```python
from build123d import *

# Parameters (mm, degrees)
SALIENTE_EXTRUIR1_DEPTH = 40
REDONDEO3_R             = 4
CROQUIS4_R              = 2.25
CORTAR_EXTRUIR3_DEPTH   = 70.282032303
CROQUIS5_R              = 4.15
CORTAR_EXTRUIR4_DEPTH   = 25
CORTAR_EXTRUIR6_DEPTH   = 1
CROQUIS9_R              = 2.65
CORTAR_EXTRUIR7_DEPTH   = 24
SALIENTE_EXTRUIR2_DEPTH = 5
SALIENTE_EXTRUIR3_START = 6
CROQUIS12_W             = 6
CROQUIS12_H             = 1.5
SALIENTE_EXTRUIR3_DEPTH = 6


with BuildPart() as part:
    # Croquis1 → Saliente-Extruir1 (new body)
    with BuildSketch(Plane(origin=(0, 0, 0), x_dir=(1, 0, 0), z_dir=(0, 1, 0))):
        Polygon((0, 0), (40, 0), (40, 20), (20, 20), (20, 40), (0, 40), align=None)
    extrude(amount=SALIENTE_EXTRUIR1_DEPTH)

    # Redondeo3
    redondeo3_edges = [part.edges().sort_by_distance(p)[0] for p in [
        (40, 40, -10),
        (0, 20, -40),
        (20, 20, -40),
        (20, 20, -20),
        (40, 20, -20),
        (40, 20, 0),
        (0, 20, 0),
        (30, 40, -20),
        (20, 40, -30),
        (10, 40, -40),
        (0, 40, -20),
        (20, 40, 0),
    ]]
    fillet(redondeo3_edges, radius=REDONDEO3_R)

    # Croquis4 → Cortar-Extruir3 (cut, through all)
    with BuildSketch(Plane(origin=(0, 40, 0), x_dir=(1, 0, 0), z_dir=(0, 1, 0))):
        with Locations(Location((10, 30, 0), (0, 0, 270))):
            Circle(CROQUIS4_R)
        with Locations(Location((10, 10, 0), (0, 0, 270))):
            Circle(CROQUIS4_R)
    extrude(amount=-CORTAR_EXTRUIR3_DEPTH, mode=Mode.SUBTRACT)

    # Croquis5 → Cortar-Extruir4 (cut)
    with BuildSketch(Plane(origin=(40, 0, 0), x_dir=(0, 0, -1), z_dir=(1, 0, 0))):
        with Locations((10, 30)):
            Circle(CROQUIS5_R)
    extrude(amount=-CORTAR_EXTRUIR4_DEPTH, mode=Mode.SUBTRACT)

    # Croquis8 → Cortar-Extruir6 (cut)
    with BuildSketch(Plane(origin=(0, 40, 0), x_dir=(1, 0, 0), z_dir=(0, 1, 0))):
        Polygon((12.421293342, 18.801682692), (12.421293342, 18.692307692), (8.267447188, 18.692307692), (8.267447188, 18), (7.652062573, 18), (7.652062573, 18.692307692), (6.267447188, 18.692307692), (6.267447188, 19.230769231), (7.652062573, 19.230769231), (7.652062573, 22.076923077), align=None)
        Polygon((8.267447188, 19.230769231), (10.873216419, 19.230769231), (8.267447188, 21.019230769), align=None, mode=Mode.SUBTRACT)
    extrude(amount=-CORTAR_EXTRUIR6_DEPTH, mode=Mode.SUBTRACT)

    # Croquis9 → Cortar-Extruir7 (cut)
    with BuildSketch(Plane.XY):
        with Locations((26, 20)):
            Circle(CROQUIS9_R)
    extrude(amount=-CORTAR_EXTRUIR7_DEPTH, mode=Mode.SUBTRACT)

    # Croquis11 → Saliente-Extruir2 (add)
    with BuildSketch(Plane(origin=(0, 40, 0), x_dir=(1, 0, 0), z_dir=(0, 1, 0))):
        with BuildLine():
            Line((30, 18.5), (39.122498999, 18.5))
            ThreePointArc((39.122498999, 18.5), (39.774254628, 17.324764885), (40, 16))
            Line((40, 16), (40, 4))
            ThreePointArc((40, 4), (39.774254628, 2.675235115), (39.122498999, 1.5))
            Line((39.122498999, 1.5), (30, 1.5))
            Line((30, 1.5), (30, 18.5))
        make_face()
    extrude(amount=-SALIENTE_EXTRUIR2_DEPTH)

    # Croquis12 → Saliente-Extruir3 (add)
    with BuildSketch(Plane(origin=(0, 40, 0), x_dir=(1, 0, 0), z_dir=(0, 1, 0)).offset(SALIENTE_EXTRUIR3_START)):
        with Locations((33, 2.25)):
            Rectangle(CROQUIS12_W, CROQUIS12_H)
        with BuildLine():
            Line((30, 18.5), (39.122498999, 18.5))
            ThreePointArc((39.122498999, 18.5), (39.57724661, 17.789778391), (39.872983346, 17))
            Line((39.872983346, 17), (30, 17))
            Line((30, 17), (30, 18.5))
        make_face()
    extrude(amount=-SALIENTE_EXTRUIR3_DEPTH)


solid = part.part
```
Here's how the part is built. I have some questions about the finished solid (model axes, mm). A direction names the side the tool comes from. Coordinates: 2 decimals unless noted, no trailing zeros. Order: outer loops, then holes, each group sorted by start corner. A loop starts at its lowest first (then second) coordinate and runs counter-clockwise, first axis right, second up.
1) Imagine slicing it at D-D on x = 26.5. List the corners of the cut face in (y, z) for me, and give its area (3 significant figures).
2) I need wall thicknesses on line 1 (X direction, y = 20, z = -10.25); line 2 (X direction, y = 16.5, z = -10); line 3 (Y direction, x = 34.75, z = -10). Which ranges of each line are inside material? Lowest first, please.
3) Will these pins go through, and if not, where does the flat tip stop? pin 1 (4 mm diameter, centred on y = 28.5, z = -11, fed in from +X); pin 2 (4 mm diameter, centred on x = 14, z = -34, fed in from +Y); pin 3 (0.8 mm diameter, centred on x = 7, y = 39.5, fed in from -Z); pin 4 (4 mm diameter, centred on x = 10, z = -30, fed in from -Y) (3 decimals).
4) Imagine slicing it at C-C on z = -10. List the corners of the cut face in (x, y) for me, and give its area (3 significant figures).
5) Imagine slicing it at A-A on y = 20. List the corners of the cut face in (x, z) for me.
6) Imagine slicing it at B-B on z = -30. List the corners of the cut face in (x, y) for me.
7) Which directions (+Z, -Z, +X, -X, +Y, -Y) give clear straight access to the entire face, cutting with the end or side of a thin tool? Please do faces 1 (the face through (27.675, 32.805, -6.941)), 2 (the face through (34, 42, -18.5)), 3 (the face through (9.59, 39.51, -20.11)).
8) We'd pull the mould along X, two halves only. Please class faces 4 (the face through (15, 30, -10)), 5 (the face through (23.353, 20.117, -9.886)), 6 (the face through (10, 18, -40)): +X half, -X half, draft (parallel to the pull), parting line (faces both ways), or undercut.
Response values:
1. outline: (0, -20) - (17.4, -20) - (17.4, 0) - (0, 0) - close; (22.6, -20) - (36, -20) arc R4 ccw to (40, -16) - (40, -4) arc R4 ccw to (36, 0) - (22.6, 0) - close; hole circle Ø8.3 at (30, -10)
1. area: 635 mm2
2. line 1: x = 0 to 7.76, 12.24 to 23.35, 28.65 to 40
2. line 2: x = 0 to 7.75, 12.25 to 40
2. line 3: y = 0 to 25.85, 34.15 to 40
3. pin 1: stops at x = 15
3. pin 2: stops at y = 40
3. pin 3: stops at z = -38.53
3. pin 4: passes through
4. outline: (0, 0) - (7.75, 0) - (7.75, 40) - (4, 40) arc R4 ccw to (0, 36) - close; (12.25, 0) - (40, 0) - (40, 25.85) - (15, 25.85) - (15, 34.15) - (40, 34.15) - (40, 40) - (12.25, 40) - close; hole circle Ø5.3 at (26, 20)
4. area: 1,190 mm2
5. outline: (0, -36) arc R4 ccw to (4, -40) - (16, -40) arc R4 ccw to (20, -36) - (20, -24) arc R4 cw to (23.35, -20.05) - (23.35, 0) - (4, 0) arc R4 ccw to (0, -4) - close; (28.65, -20) - (36, -20) arc R4 ccw to (40, -16) - (40, -4) arc R4 ccw to (36, 0) - (28.65, 0) - close; hole circle Ø4.5 at (10, -30); hole circle Ø4.5 at (10, -10)
6. outline: (0, 0) - (7.75, 0) - (7.75, 40) - (4, 40) arc R4 ccw to (0, 36) - close; (12.25, 0) - (20, 0) - (20, 36) arc R4 ccw to (16, 40) - (12.25, 40) - close
7. face 1: +X
7. face 2: -Z, +X, +Y
7. face 3: +Y
8. face 4: +X half
8. face 5: undercut
8. face 6: draft
